Source: CAD feature listing. Evaluate the final solid. Frame: model axes, mm. A direction names the side the tool comes from. Give positions to 0.01 mm unless a question says otherwise; leave off trailing zeros. Order: outer loops, then holes, each group sorted by start corner. A loop starts at its lowest first (then second) coordinate and runs counter-clockwise, first axis right, second up. Notation, with made-up numbers: M 77,49 L 111,49 A21 cw 111,78 Z; hole C 29,23.5 d3. An arc over 180 degrees is marked long. One line per question, with ' | ' between items. Start each with the question number.
from build123d import *

# Parameters (mm, degrees)
SKETCH1_R           = 5.08
BOSS_EXTRUDE1_DEPTH = 6.604
SKETCH2_R           = 6.477
CUT_EXTRUDE1_DEPTH  = 3.302
SKETCH3_R           = 75.946
SKETCH3_R_2         = 69.215
CUT_EXTRUDE2_DEPTH  = 1.27
SKETCH4_R           = 2.38125
CUT_EXTRUDE3_DEPTH  = 139.530727768
SKETCH5_R           = 3.77825
CUT_EXTRUDE4_DEPTH  = 1.27
CUT_EXTRUDE5_DEPTH  = 139.530727768
SKETCH10_R          = 57.15
SKETCH10_R_2        = 50.8
CUT_EXTRUDE6_DEPTH  = 1.27
SKETCH12_R          = 2.38125
CUT_EXTRUDE7_DEPTH  = 139.530727768
SKETCH15_R          = 3.175
CUT_EXTRUDE11_DEPTH = 1.27


with BuildPart() as part:
    # Sketch1 → Boss-Extrude1 (new body)
    with BuildSketch(Plane(origin=(0, 0, 0), x_dir=(0, 0, -1), z_dir=(1, 0, 0))):
        with BuildLine():
            Line((-65.405, -103.855072673), (65.405, -103.855072673))
            ThreePointArc((65.405, -103.855072673), (70.793153673, -101.623226346), (73.025, -96.235072673))
            Line((73.025, -96.235072673), (73.025, -69.997049759))
            ThreePointArc((73.025, -69.997049759), (74.696702219, -57.072253546), (79.601785714, -44.998103417))
            ThreePointArc((79.601785714, -44.998103417), (0, 91.44), (-79.601785714, -44.998103417))
            ThreePointArc((-79.601785714, -44.998103417), (-74.696702219, -57.072253546), (-73.025, -69.997049759))
            Line((-73.025, -69.997049759), (-73.025, -96.235072673))
            ThreePointArc((-73.025, -96.235072673), (-70.793153673, -101.623226346), (-65.405, -103.855072673))
        make_face()
        with Locations(Location((0, 0, 0), (0, 0, 180))):
            Circle(SKETCH1_R, mode=Mode.SUBTRACT)
    extrude(amount=BOSS_EXTRUDE1_DEPTH)

    # Sketch2 → Cut-Extrude1 (cut)
    with BuildSketch(Plane(origin=(0, 0, 0), x_dir=(0, 0, -1), z_dir=(1, 0, 0))):
        with Locations(Location((0, 0, 0), (0, 0, 180))):
            Circle(SKETCH2_R)
    extrude(amount=CUT_EXTRUDE1_DEPTH, mode=Mode.SUBTRACT)

    # Sketch3 → Cut-Extrude2 (cut)
    with BuildSketch(Plane(origin=(6.604, 0, 0), x_dir=(0, 0, -1), z_dir=(1, 0, 0))):
        Circle(SKETCH3_R)
        Circle(SKETCH3_R_2, mode=Mode.SUBTRACT)
    extrude(amount=-CUT_EXTRUDE2_DEPTH, mode=Mode.SUBTRACT)

    # Sketch4 → Cut-Extrude3 (cut, through all)
    with BuildSketch(Plane.ZY):
        with Locations((0, 85.09)):
            Circle(SKETCH4_R)
        with Locations((42.545, 73.690101608)):
            Circle(SKETCH4_R)
        with Locations((73.690101608, 42.545)):
            Circle(SKETCH4_R)
        with Locations((85.09, 0)):
            Circle(SKETCH4_R)
        with Locations((73.690101608, -42.545)):
            Circle(SKETCH4_R)
        with Locations((42.545, -73.690101608)):
            Circle(SKETCH4_R)
        with Locations((0, -85.09)):
            Circle(SKETCH4_R)
        with Locations((-42.545, -73.690101608)):
            Circle(SKETCH4_R)
        with Locations((-73.690101608, -42.545)):
            Circle(SKETCH4_R)
        with Locations((-85.09, 0)):
            Circle(SKETCH4_R)
        with Locations((-73.690101608, 42.545)):
            Circle(SKETCH4_R)
        with Locations((-42.545, 73.690101608)):
            Circle(SKETCH4_R)
    extrude(amount=-CUT_EXTRUDE3_DEPTH, mode=Mode.SUBTRACT)

    # Sketch5 → Cut-Extrude4 (cut)
    with BuildSketch(Plane.ZY):
        with Locations((0, 85.09)):
            Circle(SKETCH5_R)
        with Locations((42.545, 73.690101608)):
            Circle(SKETCH5_R)
        with Locations((-42.545, 73.690101608)):
            Circle(SKETCH5_R)
        with Locations((73.690101608, 42.545)):
            Circle(SKETCH5_R)
        with Locations((85.09, 0)):
            Circle(SKETCH5_R)
        with Locations((73.690101608, -42.545)):
            Circle(SKETCH5_R)
        with Locations((42.545, -73.690101608)):
            Circle(SKETCH5_R)
        with Locations((0, -85.09)):
            Circle(SKETCH5_R)
        with Locations((-42.545, -73.690101608)):
            Circle(SKETCH5_R)
        with Locations((-73.690101608, -42.545)):
            Circle(SKETCH5_R)
        with Locations((-85.09, 0)):
            Circle(SKETCH5_R)
        with Locations((-73.690101608, 42.545)):
            Circle(SKETCH5_R)
    extrude(amount=-CUT_EXTRUDE4_DEPTH, mode=Mode.SUBTRACT)

    # Sketch9 → Cut-Extrude5 (cut, through all)
    with BuildSketch(Plane.ZY):
        with BuildLine():
            Line((-8.255, 38.60465775), (-8.255, 28.191425558))
            ThreePointArc((-8.255, 28.191425558), (-9.179557622, 24.89186877), (-11.684, 22.553140447))
            ThreePointArc((-11.684, 22.553140447), (-21.997045256, 12.7), (-25.373592562, -1.157929405))
            ThreePointArc((-25.373592562, -1.157929405), (-26.146769513, -4.496204289), (-28.541990702, -6.946673071))
            Line((-28.541990702, -6.946673071), (-37.560114316, -12.153289167))
            ThreePointArc((-37.560114316, -12.153289167), (-43.454984563, -12.392041955), (-47.00205498, -7.677724445))
            ThreePointArc((-47.00205498, -7.677724445), (-41.244459855, 23.8125), (-16.851923077, 44.543835865))
            ThreePointArc((-16.851923077, 44.543835865), (-10.995669144, 43.82914153), (-8.255, 38.60465775))
        make_face()
        with BuildLine():
            Line((8.255, 38.60465775), (8.255, 28.191425558))
            ThreePointArc((8.255, 28.191425558), (9.179557622, 24.89186877), (11.684, 22.553140447))
            ThreePointArc((11.684, 22.553140447), (21.997045256, 12.7), (25.373592562, -1.157929405))
            ThreePointArc((25.373592562, -1.157929405), (26.146769513, -4.496204289), (28.541990702, -6.946673071))
            Line((28.541990702, -6.946673071), (37.560114316, -12.153289167))
            ThreePointArc((37.560114316, -12.153289167), (43.454984563, -12.392041955), (47.00205498, -7.677724445))
            ThreePointArc((47.00205498, -7.677724445), (41.244459855, 23.8125), (16.851923077, 44.543835865))
            ThreePointArc((16.851923077, 44.543835865), (10.995669144, 43.82914153), (8.255, 38.60465775))
        make_face()
        with BuildLine():
            Line((29.305114316, -26.451368583), (20.286990702, -21.244752487))
            ThreePointArc((20.286990702, -21.244752487), (16.967211891, -20.395664481), (13.689592562, -21.395211041))
            ThreePointArc((13.689592562, -21.395211041), (0, -25.4), (-13.689592562, -21.395211041))
            ThreePointArc((-13.689592562, -21.395211041), (-16.967211891, -20.395664481), (-20.286990702, -21.244752487))
            Line((-20.286990702, -21.244752487), (-29.305114316, -26.451368583))
            ThreePointArc((-29.305114316, -26.451368583), (-32.459315419, -31.437099575), (-30.150131903, -36.86611142))
            ThreePointArc((-30.150131903, -36.86611142), (0, -47.625), (30.150131903, -36.86611142))
            ThreePointArc((30.150131903, -36.86611142), (32.459315419, -31.437099575), (29.305114316, -26.451368583))
        make_face()
    extrude(amount=-CUT_EXTRUDE5_DEPTH, mode=Mode.SUBTRACT)

    # Sketch10 → Cut-Extrude6 (cut)
    with BuildSketch(Plane.ZY):
        Circle(SKETCH10_R)
        Circle(SKETCH10_R_2, mode=Mode.SUBTRACT)
    extrude(amount=-CUT_EXTRUDE6_DEPTH, mode=Mode.SUBTRACT)

    # Sketch12 → Cut-Extrude7 (cut, through all)
    with BuildSketch(Plane.ZY):
        with Locations((0, 60.874333344)):
            Circle(SKETCH12_R)
        with Locations((60.874333344, 0)):
            Circle(SKETCH12_R)
        with Locations((0, -60.874333344)):
            Circle(SKETCH12_R)
        with Locations((-60.874333344, 0)):
            Circle(SKETCH12_R)
    extrude(amount=-CUT_EXTRUDE7_DEPTH, mode=Mode.SUBTRACT)

    # Sketch15 → Cut-Extrude11 (cut)
    with BuildSketch(Plane(origin=(6.604, 0, 0), x_dir=(0, 0, -1), z_dir=(1, 0, 0))):
        with Locations((0, 60.874333344)):
            Circle(SKETCH15_R)
        with Locations((60.874333344, 0)):
            Circle(SKETCH15_R)
        with Locations((0, -60.874333344)):
            Circle(SKETCH15_R)
        with Locations((-60.874333344, 0)):
            Circle(SKETCH15_R)
    extrude(amount=-CUT_EXTRUDE11_DEPTH, mode=Mode.SUBTRACT)


solid = part.part
Item 1: Mould query, pull axis Z, two halves, no side actions, for faces 5 (the flat face through (0, -11, 1)), 6 (the cylindrical face through (3.3, 91.4, -2.7)), 7 (the cylindrical face through (3.9, -76.015, -43.061)). Classes: pulls with the +Z half, pulls with the -Z half, needs draft (parallel to the pull), parting line crosses it, or undercut.
Item 2: Cut plane C-C on z = 0. Count the separate pieces of the cut face and the enclosed holes in it, and give its area (3 significant figures).
Item 3: Reachability of faces 1 (the flat face through (1.27, -34, -38)), 2 (the flat face through (0, -48, -39)), 3 (the cylindrical face through (5.978, 0.954, 57.846)), 4 (the cylindrical face through (3.256, -20.397, -16.919)) from +Z, -Z, +X, -X, +Y, -Y: full face, straight path, thin tool, end or side. Return the list, or none.
Item 4: Cut plane A-A on y = -85.09. Return the cut outline in (x, z) (3 decimals), and give its area (3 significant figures).
Item 5: Pin query (flat end, axial travel): pin 1 Ø1 at (x, y) = (4.5, -41.5) entering from +Z; pin 2 Ø3 at (y, z) = (-1, 61.5) entering from +X; pin 3 Ø6 at (y, z) = (42.54, 73.69) entering from -X. Return the tip coordinate at first contact, or that it passes through.
Item 6: Cut plane B-B on z = -85.09. Return the cut outline in (x, y).
Item 7: Cut plane D-D on y = -53.5. Return the cut outline in (x, z).
Item 8: Line query: line 1 (Y direction, x = 0.5, z = 40); line 2 (Z direction, x = 2, y = -92) (3 decimals); line 3 (X direction, y = 66, z = 21). Output: solid intervals per line, ascending.
Results are:
1) face 5: needs draft | face 6: parting line crosses it | face 7: undercut
2) separate pieces: 7 | enclosed holes: 0 | area: 896 mm2
3) face 1: -X | face 2: +Z, -Z, -X, +Y, -Y | face 3: +X | face 4: +X, -X
4) outline: M 0,-73.025 L 6.604,-73.025 L 6.604,-2.381 L 1.27,-2.381 L 1.27,-3.778 L 0,-3.778 Z; M 0,3.778 L 1.27,3.778 L 1.27,2.381 L 6.604,2.381 L 6.604,73.025 L 0,73.025 Z | area: 930 mm2
5) pin 1: stops at z = 81.73 | pin 2: stops at x = 5.33 | pin 3: stops at x = 1.27
6) outline: M 0,-33.48 L 6.6,-33.48 L 6.6,-2.38 L 1.27,-2.38 L 1.27,-3.78 L 0,-3.78 Z; M 0,3.78 L 1.27,3.78 L 1.27,2.38 L 6.6,2.38 L 6.6,33.48 L 0,33.48 Z
7) outline: M 0,-75.78 L 6.6,-75.78 L 6.6,-53.9 L 5.33,-53.9 L 5.33,-43.91 L 6.6,-43.91 L 6.6,43.91 L 5.33,43.91 L 5.33,53.9 L 6.6,53.9 L 6.6,75.78 L 0,75.78 L 0,20.1 L 1.27,20.1 L 1.27,-20.1 L 0,-20.1 Z
8) line 1: y = -103.86 to -76.48, -70.9 to -40.82, -31.32 to -12.96, 25.85 to 31.32, 40.82 to 70.9, 76.48 to 82.23 | line 2: z = -73.025 to 73.025 | line 3: x = 0 to 5.33
